Autodesk Inventor part; units mm, degrees
ref_plane "YZ Plane" through (0, 0, 0) normal (1, 0, 0) x (0, 1, 0)
ref_plane "XZ Plane" through (0, 0, 0) normal (0, 1, 0) x (-1, 0, 0)
ref_plane "XY Plane" through (0, 0, 0) normal (0, 0, 1) x (1, 0, 0)
sketch "Sketch2" plane through (0, 0, 0) normal (0, 1, 0) x (-1, 0, 0)
  line L0 (21, 21) -> (-21, 21)
  line L1 (-21, 21) -> (-21, -21)
  line L2 (-21, -21) -> (21, -21)
  line L3 (21, -21) -> (21, 21)
  line L4 (21, 21) -> (-21, -21) construction
  line L5 (-21, 21) -> (21, -21) construction
  point P0 (0, 0)
  point P1 (-21, 0)
  dimension "d1" = 42
  dimension "d2" = 42
extrude "Extrusion1" add sketch "Sketch2" along normal blind 7.4
sketch "Sketch3" plane through (0, 7.4, 0) normal (0, 1, 0) x (1, 0, 0)
  line L0 (-10.2, -10.2) -> (10.2, -10.2)
  line L1 (10.2, -10.2) -> (10.2, 10.2)
  line L2 (10.2, 10.2) -> (-10.2, 10.2)
  line L3 (-10.2, 10.2) -> (-10.2, -10.2)
  line L4 (-10.2, -10.2) -> (10.2, 10.2) construction
  line L5 (10.2, -10.2) -> (-10.2, 10.2) construction
  line L6 (-4.612, -10.2) -> (-10.4855, -21)
  line L7 (-10.2, -4.5965) -> (-21, -12.5849)
  line L8 (-21, 21) -> (-21, -21)
  line L9 (-21, -12.5849) -> (-21, -21)
  line L10 (-21, -21) -> (-10.4855, -21)
  line L11 (-21, -21) -> (21, -21)
  line L12 (-10.2, -10.2) -> (-10.2, -4.5965)
  point P0 (0, 0)
  dimension "d5" = 20.4
  dimension "d6" = 20.4
  dimension "d9" = 5.588
extrude "Extrusion2" cut sketch "Sketch3" against normal blind 7.4
sketch "Sketch4" plane through (0, 7.4, 0) normal (0, 1, 0) x (1, 0, 0)
  circle A0 centre (0, 0) radius 13.5
  line L0 (-10.2, -4.5965) -> (-21, -12.5849)
  line L1 (-12.0945, -5.9978) -> (-21, -12.5849)
  line L2 (-21, -12.5849) -> (-21, 21)
  line L3 (-21, 21) -> (21, 21)
  line L4 (21, 21) -> (21, -21.0478)
  line L5 (-4.612, -10.2) -> (-10.4855, -21)
  line L6 (-5.7161, -12.2301) -> (-10.4855, -21)
  line L7 (-10.4855, -21) -> (21, -21)
  line L8 (21, -21) -> (-10.4855, -21)
  line L9 (10.2, 10.2) -> (10.2, -10.2)
  line L10 (8.8436, -10.2) -> (10.2, -10.2)
  line L11 (10.2, -10.2) -> (10.2, -8.8436)
  line L12 (-10.2, 10.2) -> (10.2, 10.2)
  line L13 (8.8436, 10.2) -> (10.2, 10.2)
  line L14 (10.2, 10.2) -> (10.2, 8.8436)
  line L15 (-10.2, -4.5965) -> (-10.2, 10.2)
  line L16 (-10.2, 8.8436) -> (-10.2, 10.2)
  line L17 (-10.2, 10.2) -> (-8.8436, 10.2)
  point P0 (-8.8436, 10.2)
  point P1 (10.2, -8.8436)
  dimension "d10" = 27
extrude "Extrusion3" add sketch "Sketch4" along normal blind 1 contours A0 L9 L12 L15 L0 L2 L3 L4 L7 L5 L10
fillet "Fillet4" radius 12.7 3 edges at (21, 4.2, 21) (21, 4.2, -21) (-21, 4.2, -21)
fillet "Fillet5" radius 5.08 7 edges at (-1.0927, 8.4, 21) (21, 8.4, 0) (17.2803, 8.4, -17.2803) (0, 8.4, -21) (-17.2803, 8.4, -17.2803) (-21, 8.4, 2.1424) (17.2803, 8.4, 17.2803)
fillet "Fillet6" radius 1.27 4 edges at (2.1158, 7.4, 10.2) (-10.2, 7.4, -2.1236) (0, 7.4, -10.2) (10.2, 7.4, 0)
sketch "Sketch5" plane through (0, 0, 0) normal (0, -1, 0) x (1, 0, 0)
  circle A0 centre (0, 0) radius 17
  circle A1 centre (0, 0) radius 9.6
  dimension "d19" = 34
  dimension "d20" = 19.2
extrude "Extrusion4" add sketch "Sketch5" along normal blind 13
sketch "Sketch6" plane through (0, -13, 0) normal (0, -1, 0) x (1, 0, 0)
  circle A0 centre (0, 0) radius 17
  circle A1 centre (0, 0) radius 6.5
  dimension "d23" = 13
extrude "Extrusion5" add sketch "Sketch6" along normal blind 15
sketch "Sketch8" plane through (0, -28, 0) normal (0, -1, 0) x (1, 0, 0)
  circle A0 centre (0, 0) radius 17
  circle A1 centre (0, 0) radius 3
  dimension "d29" = 6
  dimension "d32" = 34
extrude "Extrusion7" add sketch "Sketch8" along normal blind 32
properties part number "Wheel Adaptor"
Can you work these out from the model? Positions are in its coordinate system, mm. A direction names the side the tool comes from. Round coordinates to 2 decimals unless told otherwise and drop trailing zeros. Write each loop counter-clockwise with the first axis right and the second up, starting at its lowest first coordinate (ties: lowest second). Pieces come first, ordered by that corner, then holes. Notation, with made-up numbers: M 83,23 L 126,23 A25 cw 126,46 Z; hole C 52,-35.75 d10. An arc over 180 degrees is marked long. Use a Markdown table: item, result.
Item 1: For pin 1 Ø1 at (x, z) = (-12, -1) entering from +Y; pin 2 Ø10 at (x, y) = (10.5, -33.5) entering from -Z; pin 3 Ø6 at (x, y) = (6.5, -19.5) entering from +Z; pin 4 Ø5 at (x, z) = (0, 0) entering from -Y, each with a flat end and sliding along its axis, tell me the tip position at first contact or that it passes through.
Found:
| item | result |
|---|---|
| pin 1 | stops at y = 7.4 |
| pin 2 | stops at z = -16.09 |
| pin 3 | stops at z = 16.64 |
| pin 4 | passes through |
Item 2: Which directions (+Z, -Z, +X, -X, +Y, -Y) give clear straight access to the entire face, cutting with the end or side of a thin tool? Please do faces 4 (the face through (17.38, 1.64, 17.18)), 5 (the face through (1, 7.4, 12)).
Found:
| item | result |
|---|---|
| face 4 | +Z, +X, +Y, -Y |
| face 5 | +Y |
Item 3: If I drill on line 1 along Z through (x, y) = (0, -21); line 2 along Z through (x, y) = (0, -46); line 3 along Y through (x, z) = (8, -6), over which ranges is the centre line in solid material (lowest first)? Write a range as [from, to].
Found:
| item | result |
|---|---|
| line 1 | z = [-17, -6.5], [6.5, 17] |
| line 2 | z = [-17, -3], [3, 17] |
| line 3 | y = [-60, 0] |
Item 4: I want a section at D-D (y = -20). List the corners of the cut face in (x, z) for me, and give its area (3 significant figures).
Found:
| item | result |
|---|---|
| outline | C 0,0 d34; hole C 0,0 d13 |
| area | 775 mm2 |
Item 5: We'd pull the mould along Z, two halves only. Please class faces 1 (the face through (0, 2, -21)), 2 (the face through (14, 0, 10)), 3 (the face through (5.161, -6.409, -8.095)): released by +Z, released by -Z, zero draft, split by the parting line, or undercut.
Found:
| item | result |
|---|---|
| face 1 | released by -Z |
| face 2 | zero draft |
| face 3 | undercut |
Item 6: I want a section at C-C (y = -30). List the corners of the cut face in (x, z) for me, and give its area (3 significant figures).
Found:
| item | result |
|---|---|
| outline | C 0,0 d34; hole C 0,0 d6 |
| area | 880 mm2 |
